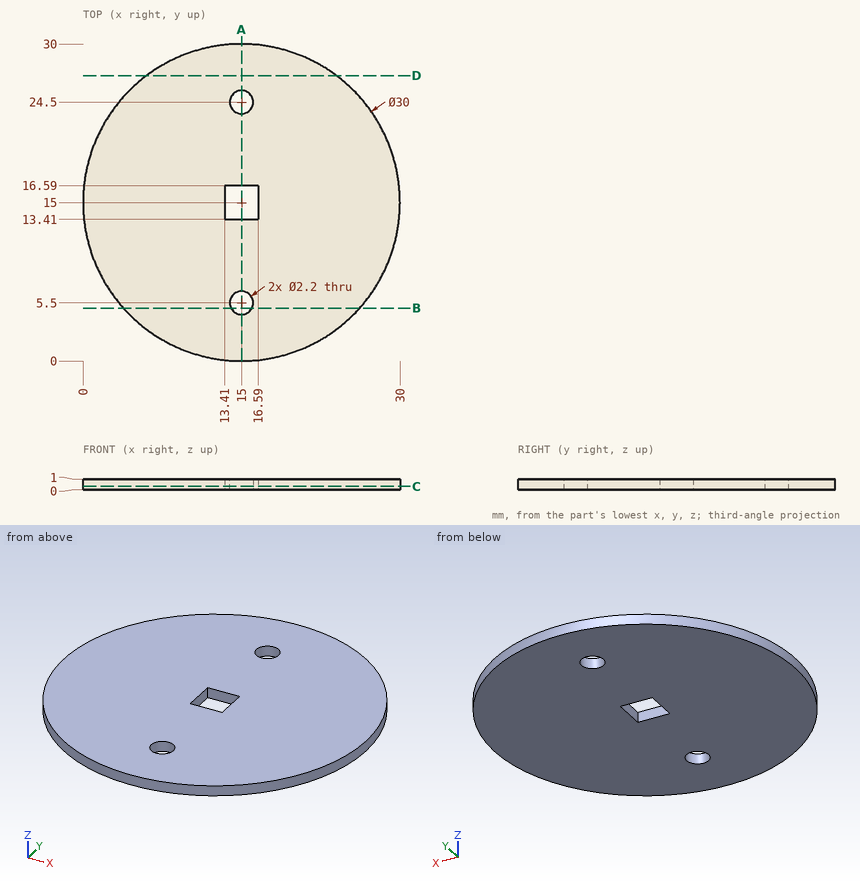
Study the drawing (mm; zero at the part's minimum x, y, z) and answer. Round coordinates to 2 decimals unless told otherwise and drop trailing zeros. Order: outer loops, then holes, each group sorted by start corner. A loop starts at its lowest first (then second) coordinate and runs counter-clockwise, first axis right, second up. Notation, with made-up numbers: (67, 42.5) -> (106, 42.5) arc R29 ccw to (106, 77.5) -> close; hole circle Ø6 at (4.5, -0.5). An arc over 180 degrees is marked (long way). Answer as CSV lines item,"result". Start each with the question number.
(1) The part is cut by section D-D (y = 27). Determine the outline of the cut face in (x, z), then the cut area to 3 significant figures.
(2) The part is cut by section A-A (x = 15). Determine the outline of the cut face in (y, z), then the cut area to 3 significant figures.
(3) The part is cut by section B-B (y = 5). Determine the outline of the cut face in (x, z), then the cut area to 3 significant figures.
(4) The part is cut by section C-C (z = 0.3). Determine the outline of the cut face in (x, y).
(5) Flat-ended cylindrical pins translate along their axes: pin 1 Ø0.5 at (x, z) = (14.5, 0.5) entering from +Y; pin 2 Ø1.3 at (x, y) = (15, 24.5) entering from +Z. Find the tip coordinate at first contact, or state that the pin passes through.
(6) Find the intervals of material crossed by probe 1 along Y at (x, z) = (15, 0.35); probe 2 along X at (y, z) = (25.5, 0.4); probe 3 along X at (y, z) = (24, 0.45), in increasing order. Write a range as from..to.
Evaluation:
1,outline,"(6, 0) -> (24, 0) -> (24, 1) -> (6, 1) -> close"
1,area,"18.0 mm²"
2,outline,"(0, 0) -> (4.4, 0) -> (4.4, 1) -> (0, 1) -> close; (6.6, 0) -> (13.41, 0) -> (13.41, 1) -> (6.6, 1) -> close; (16.59, 0) -> (23.4, 0) -> (23.4, 1) -> (16.59, 1) -> close; (25.6, 0) -> (30, 0) -> (30, 1) -> (25.6, 1) -> close"
2,area,"22.4 mm²"
3,outline,"(3.82, 0) -> (14.02, 0) -> (14.02, 1) -> (3.82, 1) -> close; (15.98, 0) -> (26.18, 0) -> (26.18, 1) -> (15.98, 1) -> close"
3,area,"20.4 mm²"
4,outline,"circle Ø30 at (15, 15); hole (13.41, 13.41) -> (16.59, 13.41) -> (16.59, 16.59) -> (13.41, 16.59) -> close; hole circle Ø2.2 at (15, 5.5); hole circle Ø2.2 at (15, 24.5)"
5,pin 1,"y = 30"
5,pin 2,"through"
6,probe 1,"0..4.4, 6.6..13.41, 16.59..23.4, 25.6..30"
6,probe 2,"4.29..14.54, 15.46..25.71"
6,probe 3,"3..14.02, 15.98..27"
